For this review, take the finished solid that the model builds, in its own axes (mm). Face numbers are marked on the shaded views. A direction names the side the tool comes from. Coordinates: 2 decimals unless noted, no trailing zeros. Write each loop counter-clockwise with the first axis right and the second up, starting at its lowest first coordinate (ties: lowest second). Pieces come first, ordered by that corner, then holes.
1) To check wall thickness, follow line 1 along Y through (x, z) = (6.5, 7.25); line 2 along Y through (x, z) = (1.5, 1.25); line 3 along Y through (x, z) = (-1, 4.5). State the ranges of each line that lie inside material, in increasing order.
2) Insertion check: P1, Ø1.5, axis at y = 0.5, z = 1, coming from the +X side; P2, Ø1.9, axis at x = 5, y = 0.5, coming from the -Z side. Each pin has a flat end and moves straight along its axis. Give the tip position at first contact, or say it passes through.
3) We need section B-B on x = 2.5. Write out the cut boundary in (y, z), then the cut area to 3 significant figures.
4) We need section C-C on y = 5.5. Give the number of separate pieces and of enclosed holes in the cut face, then the cut area to 3 significant figures.
5) For the marked faces 1 and 2, list the 3-axis set-ups (+Z, -Z, +X, -X, +Y, -Y) from which the entire face can be reached by the end or side of a thin tool; tool diameter is ignored.
6) Mouldability with a two-part tool opening along Y and no side actions: class the marked faces 3, 4, 5 and 6 as pulls with the +Y half, pulls with the -Y half, needs draft (parallel to the pull), parting line crosses it, or undercut.
7) We need section A-A on z = 1. Write out the cut boundary in (x, y).
Autodesk Inventor part; units mm, degrees
ref_plane "YZ Plane" through (0, 0, 0) normal (1, 0, 0) x (0, 1, 0)
ref_plane "XZ Plane" through (0, 0, 0) normal (0, 1, 0) x (-1, 0, 0)
ref_plane "XY Plane" through (0, 0, 0) normal (0, 0, 1) x (1, 0, 0)
sketch "Sketch1" plane through (0, 0, 0) normal (0, 0, 1) x (1, 0, 0)
  circle A0 centre (-0.7749, 5.5) radius 1
  circle A1 centre (7.2251, 5.5) radius 1
  circle A2 centre (-0.7749, -5.5) radius 1
  circle A3 centre (7.2251, -5.5) radius 1
  line L0 (11.2251, -3) -> (-3.7749, -3)
  line L1 (-3.7749, -3) -> (-3.7749, 3)
  line L2 (-3.7749, 3) -> (11.2251, 3)
  line L3 (11.2251, 3) -> (11.2251, 8)
  line L4 (11.2251, 8) -> (-8.528, 8)
  arc A4 (-8.528, -8) -> (-8.528, 8) centre (-18.7749, 0) ccw
  line L5 (-8.528, -8) -> (11.2251, -8)
  line L6 (11.2251, -8) -> (11.2251, -3)
  point P0 (0, 0)
extrude "Extrusion1" add sketch "Sketch1" along normal blind 3
sketch "Sketch2" plane through (0, 0, 3) normal (0, 0, 1) x (1, 0, 0)
  line L0 (11.2251, -8) -> (11.2251, -3)
  line L1 (11.2251, -3) -> (-3.7749, -3)
  line L2 (-3.7749, -3) -> (-3.7749, 3)
  line L3 (-3.7749, 3) -> (11.2251, 3)
  line L4 (11.2251, 3) -> (11.2251, 8)
  line L5 (11.2251, 8) -> (-8.528, 8)
  arc A0 (-8.528, -8) -> (-8.528, 8) centre (-18.7749, 0) ccw
  line L6 (-8.528, -8) -> (11.2251, -8)
  circle A1 centre (-0.7749, 5.5) radius 1
  circle A2 centre (7.2251, 5.5) radius 1
  circle A3 centre (-0.7749, -5.5) radius 1
  circle A4 centre (7.2251, -5.5) radius 1
  line L7 (11.2251, -8) -> (11.2251, -3)
  line L8 (11.2251, 3) -> (11.2251, 8)
  line L9 (11.2251, -8) -> (11.2251, 8)
  point P0 (0, 0)
extrude "Extrusion2" add sketch "Sketch2" along normal blind 5
chamfer "Chamfer1" distance 3 angle 45 1 edges at (-5.7749, 0, 8)
fillet "Fillet1" radius 1 2 edges at (-6.817, -8, 6.3872) (-6.817, 8, 6.3872)
chamfer "Chamfer2" distance 2 angle 45 1 edges at (11.2251, 0, 8)
fillet "Fillet2" radius 2 2 edges at (10.2251, -8, 7) (10.2251, 8, 7)
thicken "Thicken1" operation add thickness 0.12 both sides no extend neighbours yes toward (0, 1, 0) faces at (1.2251, 3, 1)
thicken "Thicken2" operation add thickness 0.12 both sides no extend neighbours yes toward (0, -1, 0) faces at (6.2251, -3, 1)
properties part number "armtip_2"
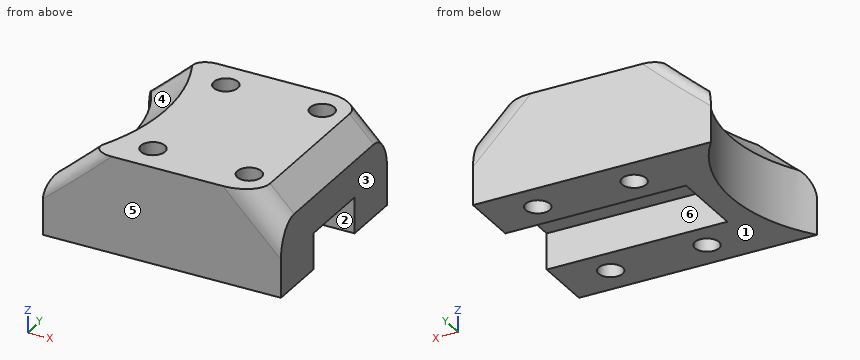
Result:
1. line 1: y = -8 to -6.19, -4.81 to 4.81, 6.19 to 8
1. line 2: y = -8 to -3.12, 3.12 to 8
1. line 3: y = -8 to -6.47, -4.53 to 4.53, 6.47 to 8
2. P1: stops at x = -3.77
2. P2: stops at z = 3
3. outline: (-8, 0) - (-3.12, 0) - (-3.12, 3) - (3.12, 3) - (3.12, 0) - (8, 0) - (8, 8) - (-8, 8) - close
3. area: 109 mm2
4. separate pieces: 3
4. enclosed holes: 0
4. area: 107 mm2
5. face 1: -Z, +X, -X, +Y, -Y
5. face 2: -Z, +X
6. face 3: needs draft
6. face 4: undercut
6. face 5: pulls with the -Y half
6. face 6: undercut
7. outline: (-8.53, -8) - (11.23, -8) - (11.23, -3.12) - (-3.77, -3.12) - (-3.77, 3.12) - (11.23, 3.12) - (11.23, 8) - (-8.53, 8) arc R13 cw to start; hole circle Ø2 at (-0.77, -5.5); hole circle Ø2 at (-0.77, 5.5); hole circle Ø2 at (7.23, -5.5); hole circle Ø2 at (7.23, 5.5)
